Source: CAD feature listing. Evaluate the final solid. Frame: model axes, mm. Face numbers are marked on the shaded views. Give positions to 0.01 mm unless a question says otherwise; leave off trailing zeros. Write each loop counter-clockwise with the first axis right and the second up, starting at its lowest first coordinate (ties: lowest second). Pieces come first, ordered by that corner, then holes. Notation, with made-up numbers: (-8.75, 81) -> (23.25, 81) arc R19 ccw to (23.25, 98) -> close; hole circle Ø5 at (69, 52). An arc over 180 degrees is marked (long way). Use one line per item in the form item = value. Start each with the question number.
(1) Draft query along Z for the marked faces 1, 2, 3 and 4. Return one class per face: pulls with the +Z half, pulls with the -Z half, needs draft (parallel to the pull), parting line crosses it, or undercut.
(2) First-contact query: P1, Ø1.5, axis at x = 22.5, z = -15, coming from the +Y side; P2, Ø3, axis at x = 24, y = -13.5, coming from the +Z side; P3, Ø6, axis at y = -13, z = -6, coming from the -X side; P4, Ø3, axis at x = 18.5, y = -4, coming from the -Z side. Flat tips, straight axial feed; report the tip coordinate or a pass-through.
(3) Material intervals for line 1 along Y through (x, z) = (20.5, -6.75); line 2 along Y through (x, z) = (19.25, -9.25); line 3 along Y through (x, z) = (25.5, -12.5), sorted ascending. Write a range as from..to.
(4) Cut plane A-A, the plane y = -10.5. Output: boundary loops of the cut face in (x, z), and give its area (3 significant figures).
(5) Cut plane B-B, the plane y = -3. Output: boundary loops of the cut face in (x, z).
Autodesk Inventor part; units mm, degrees
ref_plane "Work Plane1" through (25.296, -13.8947, -14.539) normal (-0.866, 0, 0.5) x (0.5, 0, 0.866)
ref_plane "YZ Plane" through (0, 0, 0) normal (1, 0, 0) x (0, 1, 0)
ref_plane "XZ Plane" through (0, 0, 0) normal (0, 1, 0) x (-1, 0, 0)
ref_plane "Work Plane1" through (25.296, -13.8947, -14.539) normal (-0.866, 0, 0.5) x (0.5, 0, 0.866)
sketch "Sketch1" plane through (25.296, -13.8947, -14.539) normal (-0.866, 0, 0.5) x (0.5, 0, 0.866)
  line L0 (-1.3162, -3.5246) -> (4.1688, -3.5246)
  arc A0 (-0.9285, -1.5996) -> (-0.9285, 1.1504) centre (0.3463, -0.2246) ccw
  line L1 (-0.9285, 1.1504) -> (-2.3162, 1.1504)
  line L2 (-2.3162, -1.5996) -> (-0.9285, -1.5996)
  line L3 (-1.3162, 15.5254) -> (-1.3162, 7.2404)
  line L4 (7.3438, 15.5254) -> (7.3438, -0.3496)
  arc A1 (4.1688, -3.5246) -> (7.3438, -0.3496) centre (4.1688, -0.3496) ccw
  line L5 (-1.3162, 15.5254) -> (7.3438, 15.5254)
  line L6 (-1.6912, 6.8654) -> (-2.3162, 6.8654)
  line L7 (-2.3162, -3.5246) -> (-0.9285, -3.5246)
  line L8 (-2.3162, 6.8654) -> (-2.3162, 1.1504)
  line L9 (-2.3162, -1.5996) -> (-2.3162, -3.5246)
  arc A2 (-1.6912, 6.8654) -> (-1.3162, 7.2404) centre (-1.3162, 6.8654) ccw
  point P0 (-1.3162, -1.5996)
  point P1 (-1.3162, 1.1504)
  dimension "d2" = 3.175
  dimension "d9" = 8.66
  dimension "d10" = 19.05
  dimension "d12" = 15.75
  dimension "d13" = 1.875
  dimension "d14" = 1.375
  dimension "d15" = 1.375
  dimension "d16" = 0.75
  dimension "d17" = 1
extrude "Extrusion1" add sketch "Sketch1" along normal blind 8.66
properties part number "Servo_Mount"
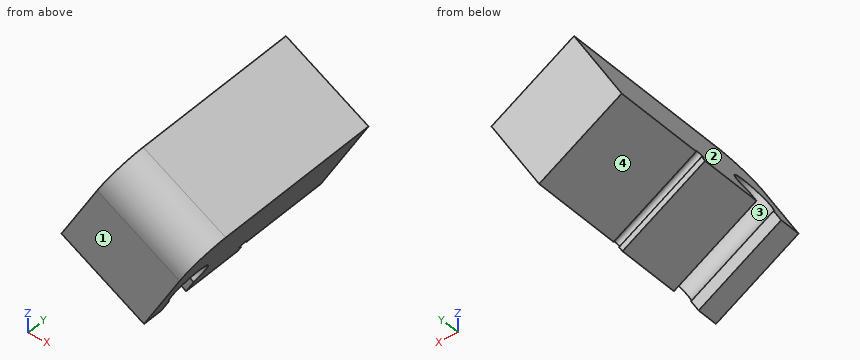
Geometry says:
q1.face_1 = needs draft
q1.face_2 = pulls with the +Z half
q1.face_3 = undercut
q1.face_4 = pulls with the -Z half
q2.P1 = 1.63
q2.P2 = -4.44
q2.P3 = 18.51
q2.P4 = -13
q3.line_1 = -17.41..1.63
q3.line_2 = -17.42..-15.55, -12.69..1.63
q3.line_3 = -17.42..-15.22, -13.02..1.63
q4.outline = (16.64, -12.21) -> (24.14, -16.54) -> (28.97, -8.18) -> (21.47, -3.85) -> close
q4.area = 83.7 mm^2
q5.outline = (17.14, -11.35) -> (24.64, -15.68) -> (28.97, -8.18) -> (21.47, -3.85) -> close
